```python
from build123d import *

# Parameters (mm, degrees)
SKETCH1_R           = 3.5
BOSS_EXTRUDE1_DEPTH = 20
SKETCH2_R           = 1
BOSS_EXTRUDE2_DEPTH = 1
SKETCH3_R           = 0.4
BOSS_EXTRUDE3_DEPTH = 5
FILLET1_R           = 0.5


with BuildPart() as part:
    # Sketch1 → Boss-Extrude1 (new body)
    with BuildSketch(Plane(origin=(0, 0, 0), x_dir=(1, 0, 0), z_dir=(0, 1, 0))):
        Circle(SKETCH1_R)
    extrude(amount=BOSS_EXTRUDE1_DEPTH)

    # Sketch2 → Boss-Extrude2 (add)
    with BuildSketch(Plane(origin=(0, 20, 0), x_dir=(1, 0, 0), z_dir=(0, 1, 0))):
        Circle(SKETCH2_R)
    extrude(amount=BOSS_EXTRUDE2_DEPTH)

    # Sketch3 → Boss-Extrude3 (add)
    with BuildSketch(Plane(origin=(0, 20, 0), x_dir=(1, 0, 0), z_dir=(0, 1, 0))):
        Circle(SKETCH3_R)
    extrude(amount=BOSS_EXTRUDE3_DEPTH)

    # Fillet1
    fillet1_edges = [part.edges().sort_by_distance(p)[0] for p in [
        (-3.5, 20, 0),
    ]]
    fillet(fillet1_edges, radius=FILLET1_R)


solid = part.part
```
For this review, take the finished solid that the model builds, in its own axes (mm). A direction names the side the tool comes from. Round coordinates to 2 decimals unless told otherwise and drop trailing zeros. Write each loop counter-clockwise with the first axis right and the second up, starting at its lowest first coordinate (ties: lowest second). Pieces come first, ordered by that corner, then holes.
1) For line 1 along Y through (x, z) = (-1, 0.5); line 2 along Y through (x, z) = (0.25, 0.5); line 3 along X through (y, z) = (23.5, 0), list the stretches that pass through material, from the lowest coordinate up.
Answer below:
line 1: y = 0 to 20
line 2: y = 0 to 21
line 3: x = -0.4 to 0.4
2) Insertion check: pin 1 Ø1.5 at (x, z) = (-1, 2) entering from +Y; pin 2 Ø3 at (x, z) = (-2, 1) entering from +Y. Each pin has a flat end and moves straight along its axis. Give the tip position at first contact, or say it passes through.
Answer below:
pin 1: stops at y = 20
pin 2: stops at y = 21
3) Take a section at C-C on y = 22. Give the boundary of the cut face in (x, z), then the cut area to 3 significant figures.
Answer below:
outline: circle Ø0.8 at (0, 0)
area: 0.503 mm2
4) Take a section at A-A on x = 0. Give the boundary of the cut face in (y, z), then the cut area to 3 significant figures.
Answer below:
outline: (0, -3.5) - (19.5, -3.5) arc R0.5 ccw to (20, -3) - (20, -1) - (21, -1) - (21, -0.4) - (25, -0.4) - (25, 0.4) - (21, 0.4) - (21, 1) - (20, 1) - (20, 3) arc R0.5 ccw to (19.5, 3.5) - (0, 3.5) - close
area: 145 mm2
5) Machinability: for faces 1 (the face through (-0.217, 20.493, 0.976)), 2 (the face through (3.233, 9.614, 1.341)), which of the approach directions +Z, -Z, +X, -X, +Y, -Y give a long, thin tool a straight path to every point of the face, cutting with its end or side? Answer none if there is none.
Answer below:
face 1: +Y
face 2: +Y, -Y
6) Take a section at B-B on z = 0. Give the boundary of the cut face in (x, y), then the cut area to 3 significant figures.
Answer below:
outline: (-3.5, 0) - (3.5, 0) - (3.5, 19.5) arc R0.5 ccw to (3, 20) - (1, 20) - (1, 21) - (0.4, 21) - (0.4, 25) - (-0.4, 25) - (-0.4, 21) - (-1, 21) - (-1, 20) - (-3, 20) arc R0.5 ccw to (-3.5, 19.5) - close
area: 145 mm2
7) Take a section at D-D on y = 10.5. Give the boundary of the cut face in (x, z), then the cut area to 3 significant figures.
Answer below:
outline: circle Ø7 at (0, 0)
area: 38.5 mm2
